```python
from build123d import *

# Parameters (mm, degrees)
SKETCH1_W                 = 55
SKETCH1_H                 = 40
SKETCH1_R                 = 17
BOSS_EXTRUDE1_DEPTH       = 20
M6_TAPPED_HOLE1_D         = 5
M6_TAPPED_HOLE1_DEPTH     = 17
M6_TAPPED_HOLE1_TIP       = 1.502151548
M4X0_7_TAPPED_HOLE3_D     = 3.3
M4X0_7_TAPPED_HOLE3_DEPTH = 12
M4X0_7_TAPPED_HOLE3_TIP   = 0.991420021


with BuildPart() as part:
    # Sketch1 → Boss-Extrude1 (new body)
    with BuildSketch(Plane.XY):
        Rectangle(SKETCH1_W, SKETCH1_H)
        Circle(SKETCH1_R, mode=Mode.SUBTRACT)
    extrude(amount=BOSS_EXTRUDE1_DEPTH)

    # M6 Tapped Hole1
    with Locations(Plane(origin=(0, 20, 0), x_dir=(1, 0, 0), z_dir=(0, 1, 0))):
        with Locations((-22.5, -10), (22.5, -10)):
            Hole(M6_TAPPED_HOLE1_D / 2, depth=M6_TAPPED_HOLE1_DEPTH)
            with Locations((0, 0, -(M6_TAPPED_HOLE1_DEPTH + M6_TAPPED_HOLE1_TIP / 2))):  # 118° drill point
                Cone(0, M6_TAPPED_HOLE1_D / 2, M6_TAPPED_HOLE1_TIP, mode=Mode.SUBTRACT)

    # M4x0.7 Tapped Hole3
    with Locations(Plane(origin=(-5.289478712, -11.13007226, 0), x_dir=(-1, 0, 0), z_dir=(0, 0, -1))):
        with Locations((-24.342037596, 0.13007226), (-24.342037596, 22.13007226), (-5.289478712, 33.13007226), (13.763080171, 22.13007226)):
            Hole(M4X0_7_TAPPED_HOLE3_D / 2, depth=M4X0_7_TAPPED_HOLE3_DEPTH)
            with Locations((0, 0, -(M4X0_7_TAPPED_HOLE3_DEPTH + M4X0_7_TAPPED_HOLE3_TIP / 2))):  # 118° drill point
                Cone(0, M4X0_7_TAPPED_HOLE3_D / 2, M4X0_7_TAPPED_HOLE3_TIP, mode=Mode.SUBTRACT)


solid = part.part
```
The listing builds one solid part. Answer for the finished solid, in the listing's coordinates (mm). A direction names the side the tool comes from. Give positions to 0.01 mm unless a question says otherwise; leave off trailing zeros. Loops run counter-clockwise (first coordinate to the right, second up) from the corner with the lowest first, then second, coordinate; pieces in that order, holes last. Notation, with made-up numbers: (46, 48.5) - (72, 48.5) arc R23 ccw to (72, 79.5) - close; hole circle Ø6 at (-26, 79.25). An arc over 180 degrees is marked (long way). Return JSON: item names as keys, results as strings. Group by question number.
1. Determine the mould class of faces 1 (the flat face through (-27.5, 0, 10)), 2 (the cylindrical face through (25, 11, 10)), 3 (the flat face through (27.5, 0, 10)) for opening direction X: pulls with the +X half, pulls with the -X half, needs draft (parallel to the pull), parting line crosses it, or undercut.
2. Find section A-A (y = 13.5). Write down the section's boundary in (x, z), then the cut area to 3 significant figures.
3. Find section C-C (x = -3). Write down the section's boundary in (y, z), then the cut area to 3 significant figures.
4. Given pin 1 Ø5 at (x, y) = (-9.5, -10) entering from -Z; pin 2 Ø3 at (x, y) = (19.05, -11) entering from -Z; pin 3 Ø3 at (x, z) = (22.5, 10) entering from +Y; pin 4 Ø2 at (x, y) = (-19.05, 11) entering from -Z, each flat-ended and moving along its own axis, determine where each tip first touches the part or whether it passes through.
5. Which of the six approach directions +Z, -Z, +X, -X, +Y, -Y give full straight-line access (tool end or side, diameter ignored) to faces 4 (the cylindrical face through (9.139, 14.334, 9.86)), 5 (the cylindrical face through (20.577, -11.632, 6.084)), 6 (the cylindrical face through (-24.81, 11.38, 10.96))?
6. Find section D-D (y = -15). Write down the section's boundary in (x, z), then the cut area to 3 significant figures.
7. Find section B-B (z = 5.25). Write down the section's boundary in (x, y).
8. Straight lines are drawn through the part: line 1 (X direction, y = 11, z = 5.5); line 2 (Y direction, x = 18.5, z = 11.75); line 3 (X direction, y = -9.5, z = 5.5). For each, find the intervals that lie inside material, in ascending order. Write a range as [from, to].
Verdict:
{
 "1": {"face 1": "pulls with the -X half", "face 2": "undercut", "face 3": "pulls with the +X half"},
 "2": {"outline": "(-27.5, 0) - (-10.33, 0) - (-10.33, 20) - (-27.5, 20) - close; (10.33, 0) - (27.5, 0) - (27.5, 20) - (10.33, 20) - close; hole circle Ø5 at (-22.5, 10); hole circle Ø5 at (22.5, 10)", "area": "647 mm^2"},
 "3": {"outline": "(-20, 0) - (-16.73, 0) - (-16.73, 20) - (-20, 20) - close; (16.73, 0) - (20, 0) - (20, 20) - (16.73, 20) - close", "area": "131 mm^2"},
 "4": {"pin 1": "passes through", "pin 2": "stops at z = 12.09", "pin 3": "stops at y = 2.4", "pin 4": "stops at z = 12.39"},
 "5": {"face 4": "+Z, -Z", "face 5": "-Z", "face 6": "+Y"},
 "6": {"outline": "(-27.5, 0) - (-8, 0) - (-8, 20) - (-27.5, 20) - close; (8, 0) - (27.5, 0) - (27.5, 20) - (8, 20) - close", "area": "780 mm^2"},
 "7": {"outline": "(-27.5, -20) - (27.5, -20) - (27.5, 20) - (-27.5, 20) - close; hole circle Ø3.3 at (-19.05, 11); hole circle Ø34 at (0, 0); hole circle Ø3.3 at (19.05, -11); hole circle Ø3.3 at (19.05, 11)"},
 "8": {"line 1": "x = [-27.5, -20.7], [-17.4, -12.96], [12.96, 17.4], [20.7, 27.5]", "line 2": "y = [-20, -12.55], [-9.45, 9.45], [12.55, 20]", "line 3": "x = [-27.5, -14.1], [14.1, 18.37], [19.74, 27.5]"}
}
